Work out the finished part from the listing and answer in its coordinate system (mm). Face numbers are marked on the shaded views. A direction names the side the tool comes from. Round coordinates to 2 decimals unless told otherwise and drop trailing zeros. Write each loop counter-clockwise with the first axis right and the second up, starting at its lowest first coordinate (ties: lowest second). Pieces come first, ordered by that corner, then holes. Notation, with made-up numbers: (17, 81.5) -> (45, 81.5) arc R4 cw to (45, 88.5) -> close; hole circle Ø10 at (37.5, 10). An arc over 180 degrees is marked (long way). One line per item, written item: value.
Autodesk Inventor part; units mm, degrees
ref_plane "YZ Plane" through (0, 0, 0) normal (1, 0, 0) x (0, 1, 0)
ref_plane "XZ Plane" through (0, 0, 0) normal (0, 1, 0) x (-1, 0, 0)
ref_plane "XY Plane" through (0, 0, 0) normal (0, 0, 1) x (1, 0, 0)
sketch "Skizze1" plane through (0, 0, 0) normal (0, 0, 1) x (1, 0, 0)
  circle A0 centre (0.0001, -0.0022) radius 3.9802
  circle A1 centre (-8.37, 7.9978) radius 1.4
  circle A2 centre (8.3745, -8.0022) radius 1.4
  line L0 (-9.5383, 7.2264) -> (-3.2198, -2.3418)
  line L1 (-7.6522, 9.1998) -> (1.8915, 3.4999)
  line L2 (9.5428, -7.2307) -> (3.3215, 2.191)
  line L3 (-1.8517, -3.5253) -> (7.6567, -9.2041)
  point P0 (0, 0)
extrude "Extrusion1" add sketch "Skizze1" along normal blind 8
sketch "Skizze2" plane through (0, 0, 8) normal (0, 0, 1) x (1, 0, 0)
  arc A0 (-7.6522, 9.1998) -> (-9.5383, 7.2264) centre (-8.37, 7.9978) ccw
  line L0 (-9.5383, 7.2264) -> (-3.2198, -2.3418)
  arc A1 (-3.2198, -2.3418) -> (-1.8517, -3.5253) centre (0.0001, -0.0022) ccw
  line L1 (-1.8517, -3.5253) -> (7.6567, -9.2041)
  arc A2 (7.6567, -9.2041) -> (9.5428, -7.2307) centre (8.3745, -8.0022) ccw
  line L2 (9.5428, -7.2307) -> (3.3215, 2.191)
  arc A3 (3.3215, 2.191) -> (1.8915, 3.4999) centre (0.0001, -0.0022) ccw
  line L3 (1.8915, 3.4999) -> (-7.6522, 9.1998)
  arc A4 (-6.6267, 10.9169) -> (-11.2072, 6.1243) centre (-8.37, 7.9978) ccw
  line L4 (-11.2072, 6.1243) -> (-4.8666, -3.4774)
  arc A5 (-4.8666, -3.4774) -> (-2.8352, -5.2674) centre (0.0001, -0.0022) ccw
  line L5 (-2.8352, -5.2674) -> (6.6312, -10.9212)
  arc A6 (6.6312, -10.9212) -> (11.2118, -6.1287) centre (8.3745, -8.0022) ccw
  line L6 (11.2118, -6.1287) -> (4.9905, 3.2931)
  arc A7 (4.9905, 3.2931) -> (2.8837, 5.2369) centre (0.0001, -0.0022) ccw
  line L7 (2.8837, 5.2369) -> (-6.6267, 10.9169)
  point P0 (0, 0)
  dimension "d2" = 2
extrude "Extrusion2" add sketch "Skizze2" against normal up to surface (8 mm away)
sketch "Skizze3" plane through (0, 0, 8) normal (0, 0, 1) x (1, 0, 0)
  circle A0 centre (0.0001, -0.0022) radius 3.9802
  circle A1 centre (-8.37, 7.9978) radius 1.4
  circle A2 centre (8.3745, -8.0022) radius 1.4
  circle A3 centre (0.0001, -0.0022) radius 2.95
  point P0 (0, 0)
  dimension "d5" = 5.9
extrude "Extrusion3" cut sketch "Skizze3" against normal through all contours A1 | A2 | A3
sketch "Skizze4" plane through (0, 0, 8) normal (0, 0, 1) x (1, 0, 0)
  circle A0 centre (-8.37, 7.9978) radius 1.4
  circle A1 centre (8.3745, -8.0022) radius 1.4
  point P0 (0, 0)
hole "Bohrung1" at (-8.37, 7.9978, 8) at (8.3745, -8.0022, 8) direction (0, 0, -1) diameter 2.8 end through all counterbore diameter 8 counterbore depth 6
properties part number "IM_Lensholder_small"
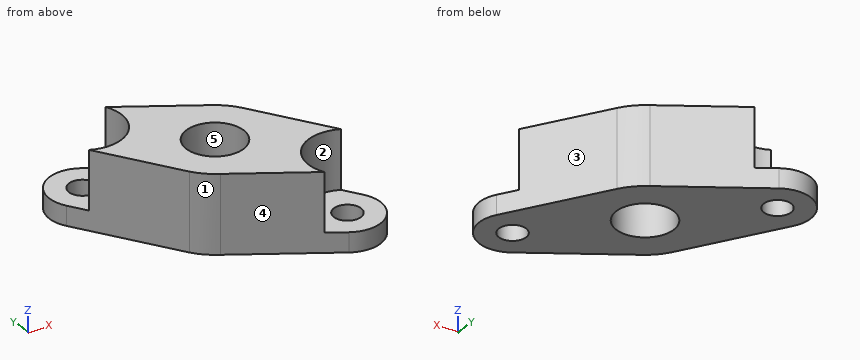
(1) For a pull along Y with two mould halves and no side action, classify the marked faces 3, 4 and 5 as pulls with the +Y half, pulls with the -Y half, needs draft (parallel to the pull), parting line crosses it, or undercut.
Reported:
face 3: pulls with the +Y half
face 4: pulls with the -Y half
face 5: undercut
(2) Find section B-B on y = -7. Give the vertices of the cut face in (x, z), plus the area to 3 significant figures.
Reported:
outline: (0.07, 0) -> (7.4, 0) -> (7.4, 2) -> (4.5, 2) -> (4.5, 8) -> (0.07, 8) -> close; (9.35, 0) -> (11.62, 0) -> (11.62, 2) -> (9.35, 2) -> close
area: 45.8 mm2
(3) Flat-ended cylindrical pins translate along their axes: pin 1 Ø2 at (x, y) = (-7, 6.5) entering from +Z; pin 2 Ø7 at (x, y) = (0, 0) entering from -Z; pin 3 Ø3 at (y, z) = (6, 2.5) entering from +X; pin 4 Ø1.5 at (x, z) = (-2.5, 3) entering from +Y. Find the tip coordinate at first contact, or state that the pin passes through.
Reported:
pin 1: stops at z = 2
pin 2: stops at z = 0
pin 3: stops at x = 3.94
pin 4: stops at y = 8.9
(4) A tool of negligible diameter and unlimited length cuts with its end or side. For the marked faces 1 and 2, from which of +Z, -Z, +X, -X, +Y, -Y can it reach the whole face along a straight path? Write none if from no direction.
Reported:
face 1: +Z, -Z, -X, -Y
face 2: +Z
(5) Find section D-D on z = 3.25. Give the vertices of the cut face in (x, y), plus the area to 3 significant figures.
Reported:
outline: (-10.05, 4.37) -> (-4.87, -3.48) arc R5.98 ccw to (-2.84, -5.27) -> (4.82, -9.84) arc R4 cw to (10.05, -4.37) -> (4.99, 3.29) arc R5.98 ccw to (2.88, 5.24) -> (-4.82, 9.84) arc R4 cw to start; hole circle Ø5.9 at (0, 0)
area: 146 mm2
(6) Find section A-A on x = 0. Give the vertices of the cut face in (y, z), plus the area to 3 significant figures.
Reported:
outline: (-6.96, 0) -> (-2.95, 0) -> (-2.95, 8) -> (-6.96, 8) -> close; (2.95, 0) -> (6.96, 0) -> (6.96, 8) -> (2.95, 8) -> close
area: 64.2 mm2
(7) Consider probe 1 along Y at (x, z) = (-0.5, 2.75); probe 2 along Z at (x, y) = (-6.75, 6); probe 3 along Y at (x, z) = (0.25, 4). Determine where each line is inside the solid, lowest interval first.
Reported:
probe 1: y = -6.66 to -2.91, 2.91 to 7.26
probe 2: z = 0 to 2
probe 3: y = -7.11 to -2.94, 2.94 to 6.81
(8) Find section C-C on z = 0.75. Give the vertices of the cut face in (x, y).
Reported:
outline: (-11.21, 6.12) -> (-4.87, -3.48) arc R5.98 ccw to (-2.84, -5.27) -> (6.63, -10.92) arc R3.4 ccw to (11.21, -6.13) -> (4.99, 3.29) arc R5.98 ccw to (2.88, 5.24) -> (-6.63, 10.92) arc R3.4 ccw to start; hole circle Ø2.8 at (-8.37, 8); hole circle Ø5.9 at (0, 0); hole circle Ø2.8 at (8.37, -8)
